Model file for the job. Use its own axes, mm. Face numbers are marked on the shaded views. A direction names the side the tool comes from. Give positions to 0.01 mm unless a question says otherwise; leave off trailing zeros. Order: outer loops, then holes, each group sorted by start corner. A loop starts at its lowest first (then second) coordinate and runs counter-clockwise, first axis right, second up. Notation, with made-up numbers: M 28,88 L 48,88 A10 cw 48,93 Z; hole C -37,80.5 d3. An arc over 180 degrees is marked long. Return JSON: item names as keys, results as strings. Group by question number.
1. 3-axis set-ups, long thin cutter, end or side, ignore diameter. For the marked faces 1 and 2: which of +Z, -Z, +X, -X, +Y, -Y reach the whole face in a straight line?
2. Slice it at D-D on x = 3.75. List the corners of the cut face in (y, z).
3. Slice it at C-C on y = 0.5. List the corners of the cut face in (x, z).
4. Slice it at A-A on x = 0. List the corners of the cut face in (y, z), then the cut area to 3 significant figures.
5. Wall check: probe 1 along X at (y, z) = (3.5, 0); probe 2 along Z at (x, y) = (0.25, 3.5); probe 3 along X at (y, z) = (-5.5, -11.25). Give the ranges that are in metal, low to high. Write a range as [from, to].
6. Two-plate mould, pull along Z, no slides. Class the marked faces 3, 4, 5 and 6: released by +Z, released by -Z, zero draft, split by the parting line, or undercut.
7. Pin check, flat tips, straight feed: pin 1 (2.5 mm diameter, centred on x = -5.46, z = 7.23, fed in from +Y); pin 2 (4 mm diameter, centred on x = 7.5, y = 2.5, fed in from +Z); pin 3 (1.5 mm diameter, centred on x = -7, y = -2.5, fed in from -Z). Stop position of each tip, or through.
8. Slice it at B-B on z = 0. List the corners of the cut face in (x, y).
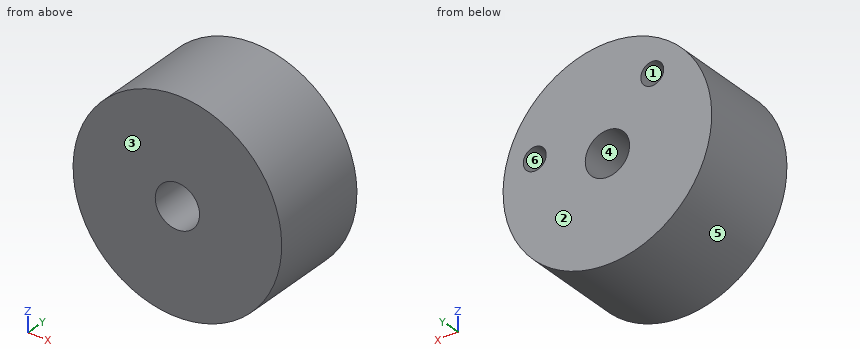
from build123d import *

# Parameters (mm, degrees)
CROQUIS1_W = 10
CROQUIS1_H = 12.5


# Read off the part's stored shape, not the designer's step: Taladro de margen para #31
with BuildPart() as part:
    # Croquis1 → Revolución1 (revolve)
    with BuildSketch(Plane.XY, mode=Mode.PRIVATE) as revoluci_n1_sk:
        with Locations((-7.7, 0)):
            Rectangle(CROQUIS1_W, CROQUIS1_H)
    revolve(revoluci_n1_sk.sketch.rotate(Axis((0, 15.597345133, 0), (0, -1, 0)), 270), axis=Axis((0, 15.597345133, 0), (0, -1, 0)))

    # Taladro de margen para #31 outline → Taladro de margen para #31 (revolve, cut)
    with BuildSketch(Plane(origin=(8.843839823, 0, 2.522833733), x_dir=(1, 0, 0), z_dir=(0, 0, 1))):
        Polygon((0, 6.25), (0, 2.410597715), (1.397, 3.25), (1.397, 6.25), align=None)
    revolve(axis=Axis((8.843839823, 0, 2.522833733), (0, 1, 0)), mode=Mode.SUBTRACT)

    # Taladro de margen para _31 2 outline → Taladro de margen para _31 2 (revolve, cut)
    with BuildSketch(Plane(origin=(-5.461397488, 0, 7.233375916), x_dir=(1, 0, 0), z_dir=(0, 0, 1))):
        Polygon((0, 6.25), (0, 2.410597715), (1.397, 3.25), (1.397, 6.25), align=None)
    revolve(axis=Axis((-5.461397488, 0, 7.233375916), (0, 1, 0)), mode=Mode.SUBTRACT)


solid = part.part
Result:
{
 "1": {"face 1": "+Y", "face 2": "+Z, -Z, +X, -X, +Y"},
 "2": {"outline": "M -6.25,-12.13 L 6.25,-12.13 L 6.25,12.13 L -6.25,12.13 Z"},
 "3": {"outline": "C 0,0 d25.4; hole C 0,0 d5.4"},
 "4": {"outline": "M -6.25,-12.7 L 6.25,-12.7 L 6.25,-2.7 L -6.25,-2.7 Z; M -6.25,2.7 L 6.25,2.7 L 6.25,12.7 L -6.25,12.7 Z", "area": "250 mm2"},
 "5": {"probe 1": "x = [-12.7, -2.7], [2.7, 12.7]", "probe 2": "z = [-12.7, -2.69], [2.69, 12.7]", "probe 3": "x = [-5.89, 5.89]"},
 "6": {"face 3": "zero draft", "face 4": "undercut", "face 5": "split by the parting line", "face 6": "undercut"},
 "7": {"pin 1": "stops at y = 3.16", "pin 2": "stops at z = 11.45", "pin 3": "stops at z = -11.06"},
 "8": {"outline": "M -12.7,-6.25 L -2.7,-6.25 L -2.7,6.25 L -12.7,6.25 Z; M 2.7,-6.25 L 12.7,-6.25 L 12.7,6.25 L 2.7,6.25 Z"}
}
